Verification items for the finished model (mm, model axes). A direction names the side the tool comes from. Coordinates: 2 decimals unless noted, no trailing zeros. Write each loop counter-clockwise with the first axis right and the second up, starting at its lowest first coordinate (ties: lowest second). Pieces come first, ordered by that corner, then holes. Notation, with made-up numbers: M 88.25,-34.75 L 134.25,-34.75 A20 cw 134.25,2.25 Z; hole C 3.25,41 d3. An arc over 180 degrees is marked long. One line per item, written item: value.
```python
from build123d import *

# Parameters (mm, degrees)
BOSS_EXTRUDE1_DEPTH = 15.24
FILLET1_R           = 12.7
SKETCH2_R           = 4.7625
CUT_EXTRUDE1_DEPTH  = 17.78
FILLET2_R           = 2.54
LPATTERN1_COUNT     = 2
LPATTERN1_PITCH     = 116.84


with BuildPart() as part:
    # Sketch1 → Boss-Extrude1 (new body)
    with BuildSketch(Plane(origin=(0, 0, 0), x_dir=(0, 0, -1), z_dir=(1, 0, 0))):
        Polygon((0, 6.35), (0, 0), (21.082, 0), (21.082, 6.35), (21.082, 84.288418695), (110.998, 84.288418695), (110.998, 0), (132.08, 0), (132.08, 6.35), (116.84, 6.35), (116.84, 97.79), (15.24, 97.79), (15.24, 6.35), align=None)
    extrude(amount=BOSS_EXTRUDE1_DEPTH)

    # Fillet1
    fillet1_edges = [part.edges().sort_by_distance(p)[0] for p in [
        (7.62, 97.79, -15.24),
        (7.62, 97.79, -116.84),
    ]]
    fillet(fillet1_edges, radius=FILLET1_R)

    # Sketch2 → Cut-Extrude1 (cut)
    with BuildSketch(Plane(origin=(0, 6.35, 0), x_dir=(1, 0, 0), z_dir=(0, 1, 0))):
        with Locations(Location((7.62, 7.62, 0), (0, 0, 270))):
            Circle(SKETCH2_R)
    cut_extrude1 = extrude(amount=-CUT_EXTRUDE1_DEPTH, mode=Mode.SUBTRACT)

    # Fillet2
    fillet2_edges = [part.edges().sort_by_distance(p)[0] for p in [
        (15.24, 84.288418695, -66.04),
        (15.24, 42.144209348, -110.998),
        (0, 42.144209348, -110.998),
        (0, 84.288418695, -66.04),
        (0, 42.144209348, -21.082),
        (7.62, 0, -21.082),
        (7.62, 84.288418695, -21.082),
        (15.24, 42.144209348, -21.082),
    ]]
    fillet(fillet2_edges, radius=FILLET2_R)

    # LPattern1: Cut-Extrude1 ×2
    with Locations(*[(0, 0, -i * LPATTERN1_PITCH) for i in range(1, LPATTERN1_COUNT)]):
        add(cut_extrude1, mode=Mode.SUBTRACT)


solid = part.part
```
Item 1: Scan lines: line 1 (X direction, y = 3.5, z = -124.46); line 2 (Z direction, x = 6.5, y = 25.5); line 3 (Y direction, x = 10.25, z = -65). Record each from-to range of solid material in increasing order.
The answers:
line 1: x = 0 to 2.86, 12.38 to 15.24
line 2: z = -116.84 to -111, -21.08 to -15.24
line 3: y = 84.29 to 97.79
Item 2: Cross-section at C-C, the plane y = 36.5. Enter the section's corners in (x, z), and give its area (3 significant figures).
The answers:
outline: M 0,-116.84 L 15.24,-116.84 L 15.24,-113.54 A2.54 ccw 12.7,-111 L 2.54,-111 A2.54 ccw 0,-113.54 Z; M 0,-18.54 A2.54 ccw 2.54,-21.08 L 12.7,-21.08 A2.54 ccw 15.24,-18.54 L 15.24,-15.24 L 0,-15.24 Z
area: 173 mm²
Item 3: Access from +Z, -Z, +X, -X, +Y, -Y to the whole of each face (thin tool, end or side, straight path). Record for faces 4 (the face through (14.516, 85.052, -69.209)), 5 (the face through (8, 45, -116.84)), 6 (the face through (8, 46, -15.24)), 7 (the face through (0.724, 42.806, -111.762)).
The answers:
face 4: +X, -Y
face 5: -Z, +X, -X, +Y
face 6: +Z, +X, -X, +Y
face 7: -X, -Y
Item 4: Cross-section at A-A, the plane z = -124.46. Enter the section's corners in (x, y).
The answers:
outline: M 0,0 L 2.86,0 L 2.86,6.35 L 0,6.35 Z; M 12.38,0 L 15.24,0 L 15.24,6.35 L 12.38,6.35 Z
Item 5: Draft check along Z on faces 1 (the face through (7.727, 0.764, -20.358)), 2 (the face through (8, 0, -13)), 3 (the face through (8, 3, 0)). Enter one of: released by +Z, released by -Z, zero draft, split by the parting line, or undercut.
The answers:
face 1: undercut
face 2: zero draft
face 3: released by +Z
Item 6: Go/stop test with flat-tipped pins: P1, Ø8, axis at x = 10, y = 44, coming from the +Z side; P2, Ø8, axis at x = 7, z = -46, coming from the -Y side; P3, Ø3, axis at x = 8, y = 32.5, coming from the -Z side. Record where each tip stops, or that it passes through.
The answers:
P1: stops at z = -15.24
P2: stops at y = 84.29
P3: stops at z = -116.84
Item 7: Cross-section at B-B, the plane x = 7.62. Enter the section's corners in (y, z), and give its area (3 significant figures).
The answers:
outline: M 0,-132.08 L 6.35,-132.08 L 6.35,-129.22 L 0,-129.22 Z; M 0,-119.7 L 6.35,-119.7 L 6.35,-116.84 L 85.09,-116.84 A12.7 ccw 97.79,-104.14 L 97.79,-27.94 A12.7 ccw 85.09,-15.24 L 6.35,-15.24 L 6.35,-12.38 L 0,-12.38 L 0,-18.54 A2.54 ccw 2.54,-21.08 L 81.75,-21.08 A2.54 cw 84.29,-23.62 L 84.29,-111 L 0,-111 Z; M 0,-2.86 L 6.35,-2.86 L 6.35,0 L 0,0 Z
area: 2,360 mm²
Item 8: Cross-section at D-D, the plane z = -65.5. Enter the section's corners in (x, y), and give its area (3 significant figures).
The answers:
outline: M 0,86.83 A2.54 ccw 2.54,84.29 L 12.7,84.29 A2.54 ccw 15.24,86.83 L 15.24,97.79 L 0,97.79 Z
area: 203 mm²
